Check sheet for the modelled part. Datum: model origin and axes. Units: mm. Face numbers are marked on the shaded views. A direction names the side the tool comes from. Give positions to 0.01 mm unless a question says otherwise; leave off trailing zeros. Order: outer loops, then holes, each group sorted by start corner. A loop starts at its lowest first (then second) coordinate and runs counter-clockwise, first axis right, second up.
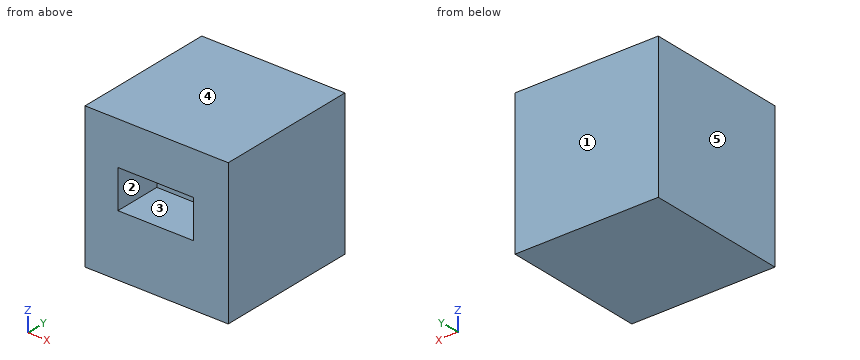
```python
from build123d import *

# Parameters (mm, degrees)
F1_W     = 76.2
F1_H     = 76.2
F2_DEPTH = 38.1
F3_W     = 40.1978772134
F3_H     = 20.4053004272
F4_DEPTH = 25.4


# Not quite as in the source:
# - a variable given as a bare number and used for a length is read in inches; the dataset says mm whatever the document's units were


with BuildPart() as f2:
    # F1 (on Front) → F2 (new body, symmetric)
    with BuildSketch(Plane.XZ):
        Rectangle(F1_W, F1_H)
    extrude(amount=F2_DEPTH, both=True)

    # F3 (on face) → F4 (cut)
    with BuildSketch(Plane.XZ.offset(38.1)):
        with Locations((-0.5212100223, 4.9419447314)):
            Rectangle(F3_W, F3_H)
    extrude(amount=-F4_DEPTH, mode=Mode.SUBTRACT)


solid = f2.part
```
(1) Gauge pin test, flat end, axial feed: pin 1 Ø6 at (x, z) = (6, 5) entering from -Y. Record the tip position at first contact, or that the pin passes through.
Response values:
pin 1: stops at y = -12.7
(2) Cross-section at B-B on z = 4.5. Enter the section's corners in (x, y), then the cut area to 3 significant figures.
Response values:
outline: (-38.1, -38.1) - (-20.62, -38.1) - (-20.62, -12.7) - (19.58, -12.7) - (19.58, -38.1) - (38.1, -38.1) - (38.1, 38.1) - (-38.1, 38.1) - close
area: 4,790 mm2
(3) Cross-section at C-C on x = 5. Enter the section's corners in (y, z).
Response values:
outline: (-38.1, -38.1) - (38.1, -38.1) - (38.1, 38.1) - (-38.1, 38.1) - (-38.1, 15.14) - (-12.7, 15.14) - (-12.7, -5.26) - (-38.1, -5.26) - close
(4) Cross-section at A-A on y = -14. Enter the section's corners in (x, z).
Response values:
outline: (-38.1, -38.1) - (38.1, -38.1) - (38.1, 38.1) - (-38.1, 38.1) - close; hole (-20.62, -5.26) - (19.58, -5.26) - (19.58, 15.14) - (-20.62, 15.14) - close
(5) Release check for a two-part mould opening along X. For the marked faces 3, 4 and 5 record: released by +X, released by -X, zero draft, split by the parting line, or undercut.
Response values:
face 3: undercut
face 4: zero draft
face 5: released by -X
(6) Set-up check for the marked faces 1 and 2: record each of +Z, -Z, +X, -X, +Y, -Y from which the full face is reachable in a straight line by a thin tool's end or side.
Response values:
face 1: +Z, -Z, +X, -X, +Y
face 2: -Y
(7) Material ranges on L1, parallel to Z at x = -4, y = -13.5; L2, parallel to X at y = -22, z = -5, recorded low to high.
Response values:
L1: z = -38.1 to -5.26, 15.14 to 38.1
L2: x = -38.1 to -20.62, 19.58 to 38.1
